from build123d import *

# Parameters (mm, degrees)
SKETCH1_W                 = 58
SKETCH1_H                 = 14
SKETCH1_R                 = 3
BOSS_EXTRUDE1_DEPTH       = 6
BOSS_EXTRUDE2_DEPTH       = 5
M4X0_7_TAPPED_HOLE1_D     = 3.3
M4X0_7_TAPPED_HOLE1_DEPTH = 9
M4X0_7_TAPPED_HOLE1_TIP   = 0.991420021
FILLET1_R                 = 6
FILLET2_R                 = 1.5
FILLET3_R                 = 0.2


with BuildPart() as part:
    # Sketch1 → Boss-Extrude1 (new body)
    with BuildSketch(Plane(origin=(0, 0, 0), x_dir=(1, 0, 0), z_dir=(0, 1, 0))):
        Rectangle(SKETCH1_W, SKETCH1_H)
        with Locations(Location((-23.71, 0, 0), (0, 0, 270))):
            Circle(SKETCH1_R, mode=Mode.SUBTRACT)
        with Locations(Location((21.29, 0, 0), (0, 0, 270))):
            Circle(SKETCH1_R, mode=Mode.SUBTRACT)
    extrude(amount=BOSS_EXTRUDE1_DEPTH)

    # Sketch2 → Boss-Extrude2 (add, symmetric)
    with BuildSketch(Plane.XY):
        with BuildLine():
            Line((12, 26), (-1.98959236, 39.202795796))
            Line((-1.98959236, 39.202795796), (-7.646446609, 33.545941546))
            Line((-7.646446609, 33.545941546), (1.899494937, 24))
            Line((1.899494937, 24), (-8, 14.100505063))
            Line((-8, 14.100505063), (-17.545941546, 23.646446609))
            Line((-17.545941546, 23.646446609), (-23.202795796, 17.98959236))
            Line((-23.202795796, 17.98959236), (-17.757359313, 12.544155877))
            ThreePointArc((-17.757359313, 12.544155877), (-16.456722805, 10.597615784), (-16, 8.30151519))
            Line((-16, 8.30151519), (-16, 6))
            Line((-16, 6), (12, 6))
            Line((12, 6), (12, 26))
        make_face()
    extrude(amount=BOSS_EXTRUDE2_DEPTH, both=True)

    # M4x0.7 Tapped Hole1
    with Locations(Plane(origin=(-20.596194078, 20.596194078, 0), x_dir=(0.7071067811865507, 0.7071067811865445, 0), z_dir=(-0.7071067811865445, 0.7071067811865507, 0))):
        with Locations((-0.686291501, 0), (23.313708499, 0)):
            Hole(M4X0_7_TAPPED_HOLE1_D / 2, depth=M4X0_7_TAPPED_HOLE1_DEPTH)
            with Locations((0, 0, -(M4X0_7_TAPPED_HOLE1_DEPTH + M4X0_7_TAPPED_HOLE1_TIP / 2))):  # 118° drill point
                Cone(0, M4X0_7_TAPPED_HOLE1_D / 2, M4X0_7_TAPPED_HOLE1_TIP, mode=Mode.SUBTRACT)

    # Fillet1
    fillet1_edges = [part.edges().sort_by_distance(p)[0] for p in [
        (12, 26, 0),
    ]]
    fillet(fillet1_edges, radius=FILLET1_R)

    # Fillet2
    fillet2_edges = [part.edges().sort_by_distance(p)[0] for p in [
        (12, 6, 0),
        (-2, 6, -5),
        (-16, 6, 0),
        (-2, 6, 5),
    ]]
    fillet(fillet2_edges, radius=FILLET2_R)

    # Fillet3
    fillet3_edges = [part.edges().sort_by_distance(p)[0] for p in [
        (29, 6, 0),
        (0, 6, -7),
        (-4.818019485, 36.374368671, -5),
        (-1.98959236, 39.202795796, 0),
        (-2.873475836, 28.772970773, -5),
        (-7.646446609, 33.545941546, 0),
        (-3.050252532, 19.050252532, -5),
        (-12.772970773, 18.873475836, -5),
        (-20.374368671, 20.818019485, -5),
        (-17.545941546, 23.646446609, 0),
        (-20.480077554, 15.266874119, -5),
        (-23.202795796, 17.98959236, 0),
        (-16.456722805, 10.597615784, -5),
        (-16, 7.900757595, -5),
        (-4.818019485, 36.374368671, 5),
        (-2.873475836, 28.772970773, 5),
        (-3.050252532, 19.050252532, 5),
        (-12.772970773, 18.873475836, 5),
        (-20.374368671, 20.818019485, 5),
        (-20.480077554, 15.266874119, 5),
        (-16.456722805, 10.597615784, 5),
        (-16, 7.900757595, 5),
        (-29, 6, 0),
        (4.064283192, 33.489399677, -5),
        (4.064283192, 33.489399677, 5),
        (11.509489653, 25.788461743, -5),
        (11.509489653, 25.788461743, 5),
        (12, 15.456215324, -5),
        (12, 15.456215324, 5),
        (-16.530926639, 6.355055975, 5.530926639),
        (12.530926639, 6.355055975, 5.530926639),
        (-16.530926639, 6.355055975, -5.530926639),
        (12.530926639, 6.355055975, -5.530926639),
        (-29, 3, -7),
        (29, 3, -7),
        (29, 3, 7),
        (-29, 3, 7),
        (0, 6, 7),
    ]]
    fillet(fillet3_edges, radius=FILLET3_R)


solid = part.part
Can you work these out from the model? Positions are in its coordinate system, mm. A direction names the side the tool comes from. Round coordinates to 2 decimals unless told otherwise and drop trailing zeros. Loops run counter-clockwise (first coordinate to the right, second up) from the corner with the lowest first, then second, coordinate; pieces in that order, holes last. Notation, with made-up numbers: (-6, -5.75) - (36, -5.75) arc R17 cw to (36, 22.25) - close; hole circle Ø6 at (21.25, 21). An arc over 180 degrees is marked (long way). Write item = value, one per line. Start each with the question number.
(1) If we section it at B-B (z = -4): Please give me the cut outline in (x, y).
(2) If we section it at A-A (x = -23.71): Please give me the cut outline in (y, z), and give its area (3 significant figures).
(3) For faces 1 (the face through (-3.08, 18.94, 4.94)), 2 (the face through (-2, 16, 5)), 3 (the face through (-3, 19.1, 0.1)), which set-ups out of +Z, -Z, +X, -X, +Y, -Y let a thin tool reach every point of the face, with its end or its side?
(4) If I drill on probe 1 along X at (y, z) = (4.45, 0); probe 2 along Y at (x, z) = (26.5, -3.5); probe 3 along Y at (x, z) = (1, -4), over which ranges is the centre line in solid material (lowest first)? Write a range as [from, to].
(5) For P1, Ø12, axis at x = -13.5, y = 9.5, coming from the +Z side; P2, Ø1, axis at y = 18, z = -0.5, coming from the -X side; P3, Ø2, axis at y = 20.5, z = -5.5, coming from the -X side; P4, Ø4, axis at x = 8.5, z = -2, coming from the +Y side, each with a flat end and sliding along its axis, tell me the tip position at first contact or that it passes through.
(6) If we mould it in two halves opening along Z, with no side actions, what happens to faces 4 (the face through (12, 15, 0)), 5 (the face through (-0.732, 34.007, -1.636)), 6 (the face through (-14.299, 13.007, 0.174)), 7 (the face through (-1.78, 6.43, 5.45))? For each: released by +Z, released by -Z, zero draft, split by the parting line, or undercut.
Ans:
q1.outline = (-29, 0) - (29, 0) - (29, 5.8) arc R0.2 ccw to (28.8, 6) - (13.5, 6) arc R1.5 cw to (12, 7.5) - (12, 23.41) arc R6 ccw to (10.12, 27.78) - (-1.85, 39.07) arc R0.2 ccw to (-2.13, 39.07) - (-7.51, 33.69) arc R0.2 ccw to (-7.51, 33.4) - (1.9, 24) - (-8, 14.1) - (-17.4, 23.51) arc R0.2 ccw to (-17.69, 23.51) - (-23.06, 18.13) arc R0.2 ccw to (-23.06, 17.85) - (-17.76, 12.54) arc R6 cw to (-16, 8.3) - (-16, 7.5) arc R1.5 cw to (-17.5, 6) - (-28.8, 6) arc R0.2 ccw to (-29, 5.8) - close
q2.outline = (0, -7) - (5.8, -7) arc R0.2 ccw to (6, -6.8) - (6, -3) - (0, -3) - close; (0, 3) - (6, 3) - (6, 6.8) arc R0.2 ccw to (5.8, 7) - (0, 7) - close
q2.area = 48.0 mm²
q3.face_1 = +Z
q3.face_2 = +Z, +X, -X, +Y
q3.face_3 = +Z, -Z
q4.probe_1 = [-29, -26.71], [-20.71, 18.29], [24.29, 29]
q4.probe_2 = [0, 6]
q4.probe_3 = [0, 23.1], [24.9, 36.38]
q5.P1 = 7
q5.P2 = -23.12
q5.P3 = -21.45
q5.P4 = 31.19
q6.face_4 = zero draft
q6.face_5 = undercut
q6.face_6 = undercut
q6.face_7 = released by +Z
